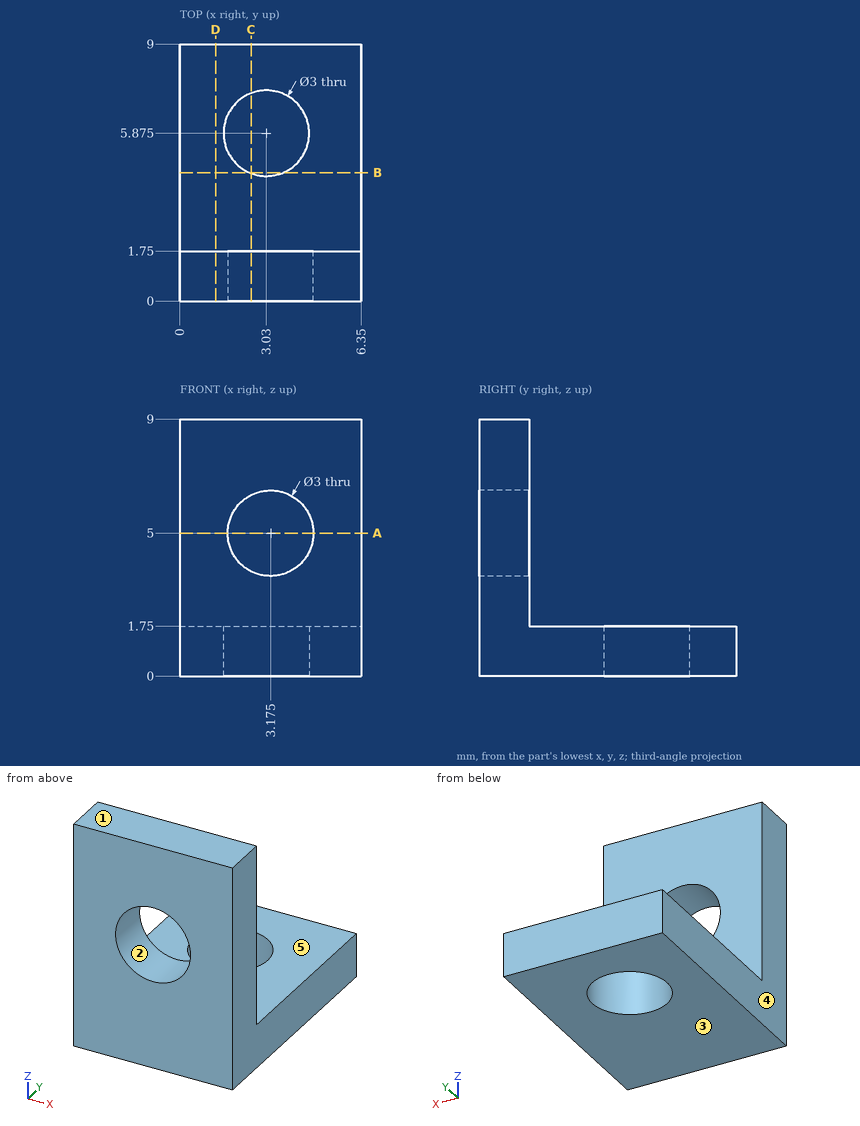
Can you work these out from the drawing? Everything is in mm from the part's minimum corner. A direction names the side the tool comes from. Round coordinates to 2 decimals unless told otherwise and drop trailing zeros. Loops run counter-clockwise (first coordinate to the right, second up) from the corner with the lowest first, then second, coordinate; pieces in that order, holes last. Notation, with made-up numbers: (69.5, 1.25) - (97.5, 1.25) arc R10 ccw to (97.5, 13.25) - close; hole circle Ø4 at (59.25, -6.5). An arc over 180 degrees is marked (long way). Answer in a Markdown table with one row per item. Add a question column.
Q1. I want a section at B-B on y = 4.5. List the corners of the cut face in (x, z) for me.
Q2. I need wall thicknesses on L1, parallel to Y at x = 3.03, z = 0.5 (3 decimals); L2, parallel to Z at x = 0.5, y = 6.5. Which ranges of each line are inside material? Lowest first, please.
Q3. I want a section at A-A on z = 5. List the corners of the cut face in (x, y) for me (3 decimals), and give its area (3 significant figures).
Q4. I want a section at C-C on x = 2.5. List the corners of the cut face in (y, z) for me, and give its area (3 significant figures).
Q5. Which directions (+Z, -Z, +X, -X, +Y, -Y) give clear straight access to the entire face, cutting with the end or side of a thin tool? Please do the marked faces 4 and 5.
Q6. We'd pull the mould along Z, two halves only. Please class the marked faces 1, 2 and 3: pulls with the +Z half, pulls with the -Z half, needs draft (parallel to the pull), parting line crosses it, or undercut.
Q7. For pin 1 Ø1.5 at (x, y) = (5, 5) entering from -Z; pin 2 Ø1.8 at (x, z) = (3.175, 5) entering from -Y; pin 3 Ø1.9 at (x, y) = (3.5, 6.5) entering from +Z, each with a flat end and sliding along its axis, tell me the tip position at first contact or that it passes through.
Q8. I want a section at D-D on x = 1.25. List the corners of the cut face in (y, z) for me, and give its area (3 significant figures).
A:
| question | item | result |
|---|---|---|
| 1 | outline | (0, 0) - (2.43, 0) - (2.43, 1.75) - (0, 1.75) - close; (3.63, 0) - (6.35, 0) - (6.35, 1.75) - (3.63, 1.75) - close |
| 2 | L1 | 0 to 4.375, 7.375 to 9 |
| 2 | L2 | 0 to 1.75 |
| 3 | outline | (0, 0) - (1.675, 0) - (1.675, 1.75) - (0, 1.75) - close; (4.675, 0) - (6.35, 0) - (6.35, 1.75) - (4.675, 1.75) - close |
| 3 | area | 5.86 mm^2 |
| 4 | outline | (0, 0) - (4.47, 0) - (4.47, 1.75) - (1.75, 1.75) - (1.75, 3.66) - (0, 3.66) - close; (0, 6.34) - (1.75, 6.34) - (1.75, 9) - (0, 9) - close; (7.28, 0) - (9, 0) - (9, 1.75) - (7.28, 1.75) - close |
| 4 | area | 18.8 mm^2 |
| 5 | face 4 | +Z, -Z, -X, +Y, -Y |
| 5 | face 5 | +Z, +X, -X, +Y |
| 6 | face 1 | pulls with the +Z half |
| 6 | face 2 | undercut |
| 6 | face 3 | pulls with the -Z half |
| 7 | pin 1 | z = 0 |
| 7 | pin 2 | through |
| 7 | pin 3 | z = 1.75 |
| 8 | outline | (0, 0) - (9, 0) - (9, 1.75) - (1.75, 1.75) - (1.75, 9) - (0, 9) - close |
| 8 | area | 28.4 mm^2 |
